The model under review builds one solid part; all positions refer to its coordinate system, in mm. Face numbers are marked on the shaded views. Round coordinates to 2 decimals unless told otherwise and drop trailing zeros. Order: outer loops, then holes, each group sorted by start corner. A loop starts at its lowest first (then second) coordinate and runs counter-clockwise, first axis right, second up. Notation, with made-up numbers: M 7.5,-9 L 61.5,-9 A15 cw 61.5,14 Z; hole C 14,-36.75 d6. An arc over 180 degrees is marked long. Answer as a JSON object with one key per item and string values. Group by question number.
1) The part is to be moulded in two halves that separate along Z. For the marked faces 1, 2, 3 and 4, say which applies: +Z half, -Z half, draft (parallel to the pull), parting line (faces both ways), or undercut.
2) Consider section B-B, the plane z = 0. Write out the cut boundary in (x, y).
3) Consider section D-D, the plane z = -15. Count the separate pieces of the cut face and the enclosed holes in it, then the cut area to 3 significant figures.
4) Consider section A-A, the plane x = 0. Write out the cut boundary in (y, z), then the cut area to 3 significant figures.
5) Consider section C-C, the plane y = -10. Write out the cut boundary in (x, z), then the cut area to 3 significant figures.
6) Insertion check: pin 1 Ø12 at (x, z) = (-33.5, 30) entering from +Y; pin 2 Ø3.5 at (x, z) = (25.98, -15) entering from -Y; pin 3 Ø8 at (x, y) = (25.5, -9.5) entering from -Z; pin 4 Ø1 at (x, y) = (35, -11.5) entering from +Z. Each pin has a flat end and moves straight along its axis. Give the tip position at first contact, or say it passes through.
7) To check wall thickness, follow line 1 (Y direction, x = 15, z = 15); line 2 (Z direction, x = 5, y = -2.25); line 3 (Z direction, x = -33.5, y = -5.5). State the ranges of each line that lie inside material, in increasing order.
```python
from build123d import *

# Parameters (mm, degrees)
SKETCH002_R        = 1.88
POCKET001_DEPTH    = 266.858481
POLARPATTERN_COUNT = 3


with BuildPart() as part:
    # Sketch → Revolution (revolve)
    with BuildSketch(Plane.XY):
        Polygon((0, 1), (35.7, 1), (44.205553, -14), (42.205553, -14), (34.7, -1), (0, -1), align=None)
    revolve(axis=Axis((0, 0, 0), (0, 1, 0)))

    # Sketch002 → Pocket001 (cut, through all)
    with BuildSketch(Plane(origin=(0, 1, 0), x_dir=(-1, 0, 0), z_dir=(0, 1, 0))):
        with Locations((0, 30)):
            Circle(SKETCH002_R)
    pocket001 = extrude(amount=-POCKET001_DEPTH, mode=Mode.SUBTRACT)

    # PolarPattern: Pocket001 ×3 about axis
    polarpattern_axis = Axis((0, 1, 0), (0, 1, 0))
    for i in range(1, POLARPATTERN_COUNT):
        add(pocket001.rotate(polarpattern_axis, i * 360 / POLARPATTERN_COUNT), mode=Mode.SUBTRACT)


solid = part.part
```
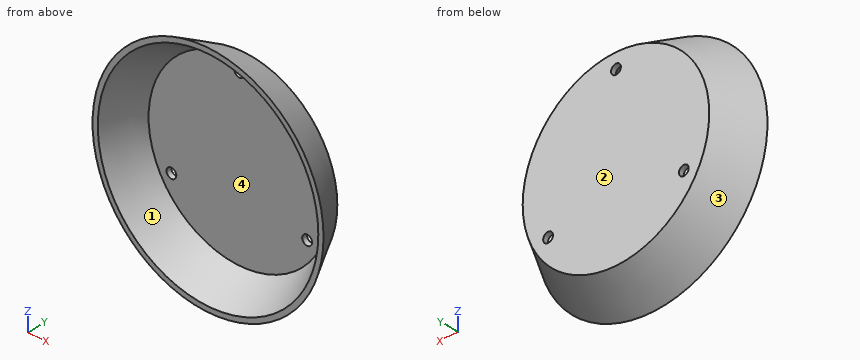
Results list:
{
 "1": {"face 1": "undercut", "face 2": "draft", "face 3": "parting line", "face 4": "undercut"},
 "2": {"outline": "M -44.21,-14 L -42.21,-14 L -34.7,-1 L 34.7,-1 L 42.21,-14 L 44.21,-14 L 35.7,1 L -35.7,1 Z"},
 "3": {"separate pieces": "3", "enclosed holes": "0", "area": "175 mm^2"},
 "4": {"outline": "M -14,-44.21 L 1,-35.7 L 1,28.12 L -1,28.12 L -1,-34.7 L -14,-42.21 Z; M -14,42.21 L -1,34.7 L -1,31.88 L 1,31.88 L 1,35.7 L -14,44.21 Z", "area": "191 mm^2"},
 "5": {"outline": "C 0,0 d83.87; hole C 0,0 d79.79", "area": "525 mm^2"},
 "6": {"pin 1": "y = -4.77", "pin 2": "through", "pin 3": "z = -36.84", "pin 4": "z = 25.46"},
 "7": {"line 1": "-1 to 1", "line 2": "-37.21 to -35.07, 35.07 to 37.21", "line 3": "-20.71 to -16.4, 16.4 to 20.71"}
}
